Check sheet for the drawn part. Datum: minimum x, y, z corner. Units: mm. A direction names the side the tool comes from. Give positions to 0.01 mm unless a question says otherwise; leave off trailing zeros. Loops run counter-clockwise (first coordinate to the right, second up) from the corner with the lowest first, then second, coordinate; pieces in that order, holes last. Notation, with made-up numbers: (54, 73.5) - (72, 73.5) arc R28 cw to (72, 110.5) - close; hole circle Ø3 at (31, -9.75). An arc over 180 degrees is marked (long way). One line per item, written item: value. Start each with the question number.
1. Sectioned sample at C-C (z = 1.35). Record the cut outline in (x, y), plus the area to 3 significant figures.
2. Access from +Z, -Z, +X, -X, +Y, -Y to the whole of each face (thin tool, end or side, straight path). Record for the marked faces 4 and 5.
3. Mould release check, pull along X, two halves, no side actions. Record for the marked faces 1, 2 and 3: pulls with the +X half, pulls with the -X half, needs draft (parallel to the pull), parting line crosses it, or undercut.
4. Sectioned sample at B-B (x = 4). Record the cut outline in (y, z).
5. Scan lines: L1, parallel to Y at x = 4, z = 1.5; L2, parallel to Z at x = 1.25, y = 3.5; L3, parallel to Y at x = 4.25, z = 3.25. Record each from-to range of solid material in increasing order. Write a range as [from, to].
6. Gauge pin test, flat ends, axial feed: pin 1 (2 mm diameter, centred on x = 2.5, z = 2, fed in from -Y); pin 2 (1.8 mm diameter, centred on x = 5.5, y = 5, fed in from +Z). Record the tip position at first contact, or that the pin passes through.
7. Sectioned sample at A-A (z = 3.65). Record the cut outline in (x, y).
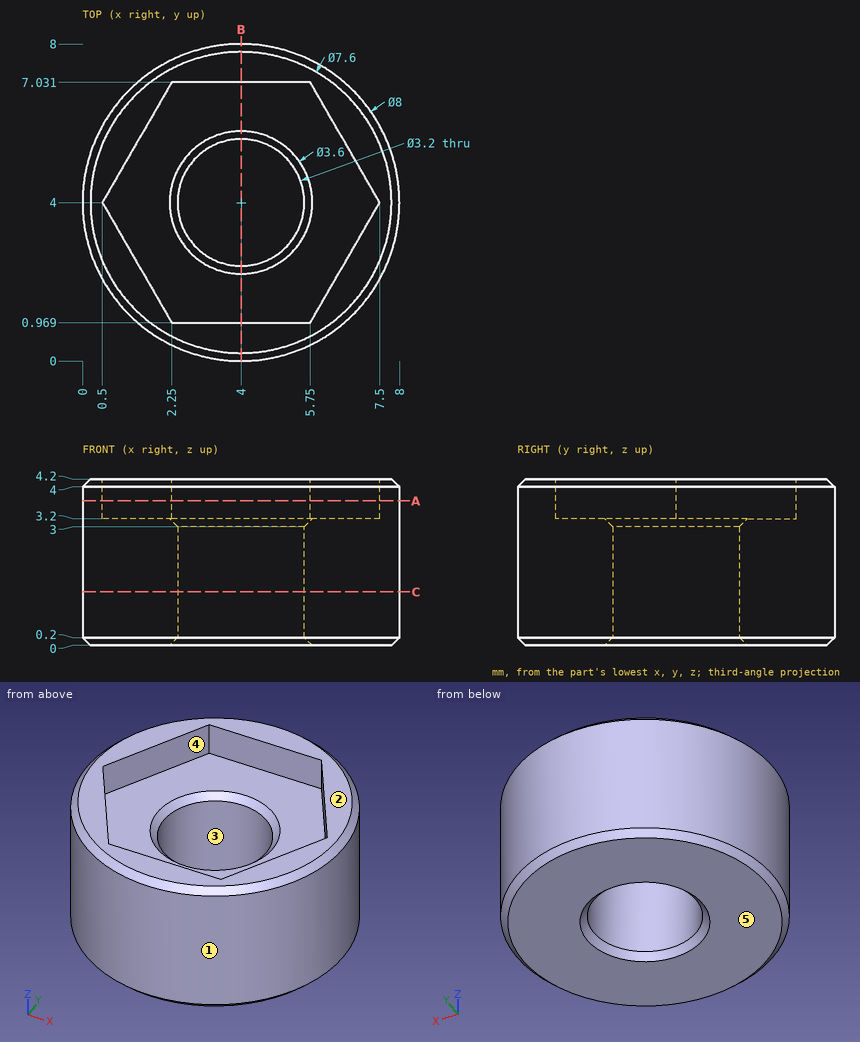
Results are:
1. outline: circle Ø8 at (4, 4); hole circle Ø3.2 at (4, 4)
1. area: 42.2 mm^2
2. face 4: +Z
2. face 5: -Z, +X, -X, +Y, -Y
3. face 1: parting line crosses it
3. face 2: needs draft
3. face 3: undercut
4. outline: (0, 0.2) - (0.2, 0) - (2.2, 0) - (2.4, 0.2) - (2.4, 3) - (2.2, 3.2) - (0.97, 3.2) - (0.97, 4.2) - (0.2, 4.2) - (0, 4) - close; (5.6, 0.2) - (5.8, 0) - (7.8, 0) - (8, 0.2) - (8, 4) - (7.8, 4.2) - (7.03, 4.2) - (7.03, 3.2) - (5.8, 3.2) - (5.6, 3) - close
5. L1: y = [0, 2.4], [5.6, 8]
5. L2: z = [0, 3.2]
5. L3: y = [0.01, 0.97], [7.03, 7.99]
6. pin 1: stops at y = 0.03
6. pin 2: stops at z = 3.2
7. outline: circle Ø8 at (4, 4); hole (0.5, 4) - (2.25, 0.97) - (5.75, 0.97) - (7.5, 4) - (5.75, 7.03) - (2.25, 7.03) - close
